For this review, take the finished solid that the model builds, in its own axes (mm). Face numbers are marked on the shaded views. A direction names the side the tool comes from. Coordinates: 2 decimals unless noted, no trailing zeros. Order: outer loops, then holes, each group sorted by start corner. A loop starts at its lowest first (then second) coordinate and runs counter-clockwise, first axis right, second up.
from build123d import *

# Parameters (mm, degrees)
BOSS_EXTRUDE1_DEPTH      = 20
SHELL1_T                 = -5
SHELL1_THICKNESS_2_DEPTH = 3
BOSS_EXTRUDE2_DEPTH      = 10
SKETCH7_W                = 23
SKETCH7_H                = 13
CUT_EXTRUDE1_DEPTH       = 8
SKETCH8_R                = 6.5
CUT_EXTRUDE2_DEPTH       = 8
SKETCH9_R                = 1
CUT_EXTRUDE3_DEPTH       = 8
SKETCH10_R               = 2.5
SKETCH10_R_2             = 1
CUT_EXTRUDE4_DEPTH       = 8
FILLET1_R                = 5


with BuildPart() as part:
    # Sketch2 → Boss-Extrude1 (new body)
    with BuildSketch(Plane(origin=(0, 0, 0), x_dir=(1, 0, 0), z_dir=(0, 1, 0))):
        with BuildLine():
            Line((0, 0), (0, 44.78))
            Line((0, 44.78), (51.787964706, 43.876037714))
            ThreePointArc((51.787964706, 43.876037714), (63.268632411, 38.943553604), (68, 27.378550743))
            Line((68, 27.378550743), (68, 17.401449257))
            ThreePointArc((68, 17.401449257), (63.268632411, 5.836446396), (51.787964706, 0.903962286))
            Line((51.787964706, 0.903962286), (0, 0))
        make_face()
    extrude(amount=BOSS_EXTRUDE1_DEPTH)

    # Shell1
    shell1_openings = [part.faces().sort_by_distance(p)[0] for p in [
        (32.484056968, 20, -22.39),
    ]]
    offset(amount=SHELL1_T, openings=shell1_openings, kind=Kind.INTERSECTION)

    # Shell1 thickness 2 face (on inner face of the shell) → Shell1 thickness 2 (cut)
    with BuildSketch(Plane(origin=(32.938254764, 5, -22.39), x_dir=(0, 0, -1), z_dir=(0, -1, 0))):
        with BuildLine():
            Line((-17.301963035, -27.938254764), (-16.486799238, 18.76244791))
            ThreePointArc((-16.486799238, 18.76244791), (-13.049007283, 26.764125401), (-4.988550743, 30.061745236))
            Line((-4.988550743, 30.061745236), (4.988550743, 30.061745236))
            ThreePointArc((4.988550743, 30.061745236), (13.049007283, 26.764125401), (16.486799238, 18.76244791))
            Line((16.486799238, 18.76244791), (17.301963035, -27.938254764))
            Line((17.301963035, -27.938254764), (-17.301963035, -27.938254764))
        make_face()
    extrude(amount=SHELL1_THICKNESS_2_DEPTH, mode=Mode.SUBTRACT)

    # Sketch6 → Boss-Extrude2 (add)
    with BuildSketch(Plane(origin=(0, 2, 0), x_dir=(1, 0, 0), z_dir=(0, 1, 0))):
        with BuildLine():
            Line((23, 39.377771866), (23, 5.402228134))
            Line((23, 5.402228134), (51.700702674, 5.903200762))
            ThreePointArc((51.700702674, 5.903200762), (59.702380165, 9.340992717), (63, 17.401449257))
            Line((63, 17.401449257), (63, 27.378550743))
            ThreePointArc((63, 27.378550743), (59.702380165, 35.439007283), (51.700702674, 38.876799238))
            Line((51.700702674, 38.876799238), (23, 39.377771866))
        make_face()
    extrude(amount=BOSS_EXTRUDE2_DEPTH)

    # Sketch7 → Cut-Extrude1 (cut)
    with BuildSketch(Plane(origin=(0, 12, 0), x_dir=(1, 0, 0), z_dir=(0, 1, 0))):
        with Locations((45, 22.39)):
            Rectangle(SKETCH7_W, SKETCH7_H)
    extrude(amount=-CUT_EXTRUDE1_DEPTH, mode=Mode.SUBTRACT)

    # Sketch8 → Cut-Extrude2 (cut)
    with BuildSketch(Plane(origin=(0, 4, 0), x_dir=(1, 0, 0), z_dir=(0, 1, 0))):
        with Locations(Location((50, 22.39, 0), (0, 0, 90))):
            Circle(SKETCH8_R)
    extrude(amount=-CUT_EXTRUDE2_DEPTH, mode=Mode.SUBTRACT)

    # Sketch9 → Cut-Extrude3 (cut)
    with BuildSketch(Plane(origin=(0, 12, 0), x_dir=(1, 0, 0), z_dir=(0, 1, 0))):
        with Locations(Location((31.2, 22.39, 0), (0, 0, 270))):
            Circle(SKETCH9_R)
        with Locations(Location((58.8, 22.39, 0), (0, 0, 270))):
            Circle(SKETCH9_R)
    extrude(amount=-CUT_EXTRUDE3_DEPTH, mode=Mode.SUBTRACT)

    # Sketch10 → Cut-Extrude4 (cut)
    with BuildSketch(Plane(origin=(5, 0, 0), x_dir=(0, 0, -1), z_dir=(1, 0, 0))):
        with Locations((22.39, 10)):
            Circle(SKETCH10_R)
        with Locations((17.89, 10)):
            Circle(SKETCH10_R_2)
        with Locations((26.89, 10)):
            Circle(SKETCH10_R_2)
    extrude(amount=-CUT_EXTRUDE4_DEPTH, mode=Mode.SUBTRACT)

    # Fillet1
    fillet1_edges = [part.edges().sort_by_distance(p)[0] for p in [
        (68, 20, -22.39),
        (63.268632411, 20, -38.943553604),
        (25.893982353, 20, -44.328018857),
        (23, 12, -22.39),
        (25.893982353, 20, -0.451981143),
        (25.893982353, 0, -44.328018857),
        (63.268632411, 0, -38.943553604),
        (68, 0, -22.39),
        (63.268632411, 0, -5.836446396),
        (25.893982353, 0, -0.451981143),
        (63.268632411, 20, -5.836446396),
    ]]
    fillet(fillet1_edges, radius=FILLET1_R - 0.0001)  # a hair under: the kernel refuses the full size


solid = part.part
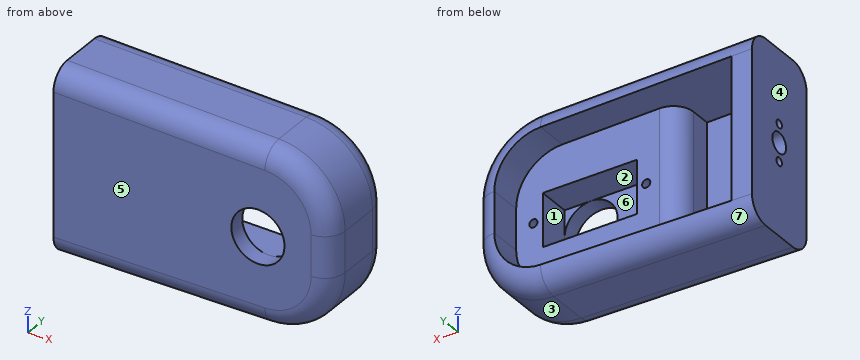
1. Take a section at A-A, the plane y = 10. Give the boundary of the cut face in (x, z), plus the area to 3 significant figures.
Answer below:
outline: (0, -44.78) - (51.79, -43.88) arc R16.5 ccw to (68, -27.38) - (68, -17.4) arc R16.5 ccw to (51.79, -0.9) - (0, 0) - (0, -16.89) - (5, -16.89) - (5, -5.09) - (24, -5.42) - (24, -39.36) - (5, -39.69) - (5, -27.89) - (0, -27.89) - close; (0, -25.89) - (5, -25.89) - (5, -24.89) - (0, -24.89) - close; (0, -19.89) - (5, -19.89) - (5, -18.89) - (0, -18.89) - close; hole circle Ø2 at (31.2, -22.39); hole (33.5, -28.89) - (56.5, -28.89) - (56.5, -15.89) - (33.5, -15.89) - close; hole circle Ø2 at (58.8, -22.39)
area: 1,850 mm2
2. Take a section at B-B, the plane y = 17.75. Give the boundary of the cut face in (x, z).
Answer below:
outline: (0, -43.96) - (51.77, -43.05) arc R15.68 ccw to (67.18, -27.38) - (67.18, -17.4) arc R15.68 ccw to (51.77, -1.73) - (0, -0.82) - close; hole (5, -39.69) - (51.7, -38.88) arc R11.5 ccw to (63, -27.38) - (63, -17.4) arc R11.5 ccw to (51.7, -5.9) - (5, -5.09) - close
3. To check wall thickness, follow L1, parallel to X at y = 8, z = -22.39; L2, parallel to Y at x = 30.5, z = -25; L3, parallel to Y at x = 21, z = -14. State the ranges of each line that lie inside material, in increasing order.
Answer below:
L1: x = 23.1 to 30.2, 32.2 to 33.5, 56.5 to 57.8, 59.8 to 68
L2: y = 0 to 12
L3: y = 0 to 2
4. Machinability: for the marked faces 5, 6 and 7, which of the approach directions +Z, -Z, +X, -X, +Y, -Y give a long, thin tool a straight path to every point of the face, cutting with its end or side? Answer none if there is none.
Answer below:
face 5: +Z, -Z, +X, -X, -Y
face 6: +Y
face 7: -Z, +X, +Y
5. Clearance check with flat-ended pins moving along their axes: pin 1 Ø9 at (x, y) = (45, 6.5) entering from +Z; pin 2 Ø10 at (x, y) = (22.5, 17) entering from +Z; pin 3 Ø9 at (x, y) = (41, 9) entering from -Z. State where each tip first meets the part, or that it passes through.
Answer below:
pin 1: stops at z = -0.71
pin 2: stops at z = -0.31
pin 3: stops at z = -44.14
6. The part is to be moulded in two halves that separate along X. For the marked faces 1, 2, 3 and 4, say which applies: +X half, -X half, draft (parallel to the pull), parting line (faces both ways), or undercut.
Answer below:
face 1: undercut
face 2: undercut
face 3: +X half
face 4: -X half
